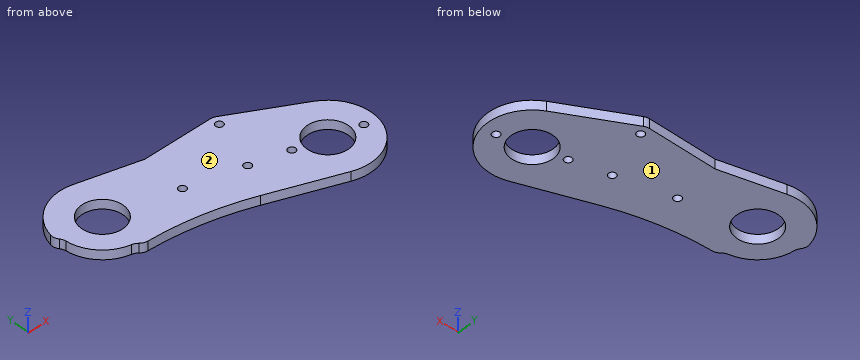
Autodesk Inventor part; units mm, degrees
ref_plane "YZ Plane" through (0, 0, 0) normal (1, 0, 0) x (0, 1, 0)
ref_plane "XZ Plane" through (0, 0, 0) normal (0, 1, 0) x (-1, 0, 0)
ref_plane "XY Plane" through (0, 0, 0) normal (0, 0, 1) x (1, 0, 0)
sketch "Sketch1" plane through (0, 0, 0) normal (0, 0, 1) x (1, 0, 0)
  circle A0 centre (71.842, 71.842) radius 50.8 construction
  circle A1 centre (-71.842, -71.842) radius 50.8 construction
  circle A2 centre (0, 0) radius 50.8 construction
  line L0 (-35.921, -35.921) -> (35.921, 35.921) construction
  line L1 (71.842, 71.842) -> (-71.842, -71.842) construction
  line L2 (-4.3707, 6.2419) -> (-4.3707, 50.6116) construction
  line L3 (-226.8798, -122.642) -> (638.5123, -122.642) construction
  circle A3 centre (147.8406, -65.492) radius 57.15 construction
  circle A4 centre (71.842, 71.842) radius 14.2621
  circle A5 centre (-71.842, -71.842) radius 14.2621
  circle A6 centre (-4.3707, 6.2419) radius 57.15 construction
  circle A7 centre (-71.842, -71.842) radius 30.1371 construction
  circle A8 centre (71.842, 71.842) radius 30.1371 construction
  circle A9 centre (-56.3286, 101.6778) radius 14.2621
  line L4 (-56.3286, 101.6778) -> (71.842, 71.842) construction
  circle A10 centre (71.842, 71.842) radius 14.3256 construction
  circle A11 centre (-71.842, -71.842) radius 14.3256 construction
  circle A12 centre (-78.675, 59.5778) radius 14.2621
  line L5 (-71.842, -71.842) -> (-78.675, 59.5778) construction
  circle A13 centre (-78.675, 59.5778) radius 23.8316 construction
  circle A14 centre (-56.3286, 101.6778) radius 23.8316 construction
  line L6 (14.7165, 60.1103) -> (61.7767, 43.4355)
  line L7 (-43.0113, -63.0652) -> (-59.0434, -10.4018)
  arc A15 (14.7165, 60.1103) -> (-59.0434, -10.4018) centre (-4.3707, 6.2419) ccw
  line L8 (-202.9564, 165.4321) -> (-177.9423, 161.0215)
  line L9 (-177.9423, 161.0215) -> (-204.4062, 10.9368) construction
  line L10 (-204.4062, 10.9368) -> (-229.4204, 15.3474) construction
  line L11 (-229.4204, 15.3474) -> (-202.9564, 165.4321) construction
  line L12 (-248.4004, -92.2937) -> (35.0702, -142.2772) construction
  line L13 (-201.8537, 171.6857) -> (161.0026, 107.7043) construction
  line L14 (-201.8537, 171.6857) -> (-248.4004, -92.2937) construction
  circle A16 centre (-147.7392, 94.6182) radius 31.75 construction
  line L15 (-77.4376, 35.7784) -> (-74.4797, -21.1106) construction
  line L16 (-190.4493, 163.2268) -> (-216.9133, 13.1421) construction
  line L17 (-193.206, 147.593) -> (-214.1566, 28.7759) construction
  circle A17 centre (-147.7392, 94.6182) radius 17.4625 construction
  circle A18 centre (-147.7392, 94.6182) radius 9.525
  circle A19 centre (-56.3286, 101.6778) radius 30.1816 construction
  line L18 (-202.9564, 165.4321) -> (-229.4204, 15.3474)
  arc A20 (61.7767, 43.4355) -> (78.6846, 101.1921) centre (71.842, 71.842) ccw
  arc A21 (-99.1524, -84.5852) -> (-43.0113, -63.0652) centre (-71.842, -71.842) ccw
  line L19 (-147.7392, 94.6182) -> (-131.3298, 100.5908) construction
  line L20 (-113.4287, 107.1063) -> (-182.0497, 82.1302) construction
  circle A22 centre (-182.0497, 82.1302) radius 4.7625 construction
  line L21 (0, 0) -> (-4.3707, 6.2419) construction
  circle A23 centre (71.842, 71.842) radius 28.6512 construction
  line L22 (62.334, 44.8145) -> (-61.0615, 88.2239) construction
  line L23 (75.2477, 100.2901) -> (-54.6333, 115.8388) construction
  line L24 (-177.9423, 161.0215) -> (78.6846, 101.1921)
  line L25 (-147.7392, 94.6182) -> (-125.7265, 22.8485) construction
  circle A24 centre (-125.7265, 22.8485) radius 31.75 construction
  circle A25 centre (-125.7265, 22.8485) radius 14.2621
  line L26 (-78.675, 59.5778) -> (-125.7265, 22.8485) construction
  circle A26 centre (-147.7392, 94.6182) radius 25.4 construction
  arc A27 (-99.1524, -84.5852) -> (-229.4204, 15.3474) centre (-260.2996, -159.7777) ccw
  circle A28 centre (-147.7392, 94.6182) radius 36.5125 construction
  line L27 (-180.8308, 110.0491) -> (-147.7392, 94.6182) construction
  arc A29 (-39.1085, 126.4648) -> (-49.6289, 131.1064) centre (-56.3286, 101.6778) ccw
  arc A30 (-38.1634, 52.3307) -> (-39.1085, 126.4648) centre (-65.0941, 89.0604) ccw
  arc A31 (14.7165, 60.1103) -> (-55.7287, 71.5022) centre (-51.7719, -127.535) ccw
  arc A32 (-49.6289, 131.1064) -> (-55.7287, 71.5022) centre (-56.3286, 101.6778) ccw
  line L28 (-10.7972, 91.0789) -> (26.3107, 82.4409) construction
  point P0 (-75.9587, 7.3339)
  point P1 (-203.6813, 88.1845)
  point P2 (-203.6813, 88.1845)
  point P3 (-144.7069, 111.8154)
  point P4 (-161.1163, 105.8429)
  point P5 (-164.1486, 88.6457)
  point P6 (-150.7715, 77.421)
  point P7 (-134.3622, 83.3936)
  point P8 (-123.871, 103.3056)
  point P9 (-143.3285, 119.6324)
  point P10 (-167.1967, 110.945)
  point P11 (-171.6074, 85.9309)
  point P12 (-152.1499, 69.6041)
  point P13 (-128.2817, 78.2914)
  point P14 (-160.2272, 128.9288)
  point P15 (-182.0497, 82.1302)
  point P16 (-135.2512, 60.3077)
  point P17 (-132.3084, 127.7098)
  point P18 (-163.1701, 61.5267)
  point P19 (-114.6476, 79.1874)
  point P20 (-49.4759, 131.0711)
  point P21 (7.7567, 86.7599)
  dimension "d7" = 101.6
  dimension "d18" = 47.6631
  dimension "d34" = 34.925
  dimension "d65" = 50.8
  dimension "d3" = 45
  dimension "d4" = 0
  dimension "d8" = 101.6
  dimension "d9" = 28.5242
  dimension "d10" = 101.6
  dimension "d11" = 114.3
  dimension "d12" = 114.3
  dimension "d13" = 15.875
  dimension "d14" = 15.875
  dimension "d15" = 131.5974
  dimension "d16" = 28.6512
  dimension "d17" = 131.5974
  dimension "d19" = 47.6631
  dimension "d22" = 25.4
  dimension "d23" = 152.4
  dimension "d26" = 268.0517
  dimension "d27" = 63.5
  dimension "d30" = 203.2
  dimension "d31" = 10
  dimension "d33" = 120.65
  dimension "d35" = 19.05
  dimension "d36" = 6.35
  dimension "d40" = 360
  dimension "d44" = 9.525
  dimension "d55" = 80
  dimension "d56" = 7.62
  dimension "d57" = 6.35
  dimension "d58" = 57.3024
  dimension "d59" = 63.5
  dimension "d60" = 75.0697
  dimension "d61" = 59.69
  dimension "d62" = 55
  dimension "d68" = 360
  dimension "d70" = 41.275
  dimension "d71" = 60
  dimension "d82" = 360
  dimension "d87" = 360
  dimension "d89" = 45
  dimension "d105" = 38.1
extrude "Extrusion1" add sketch "Sketch1" along normal blind 6.35 contours A29 A30 A31 A32 | A31 A30 A29 L24 A20 L6
hole "Hole1" at (-193.206, 147.593, 0) at (-203.6813, 88.1845, 0) at (-214.1566, 28.7759, 0) at (-131.3298, 100.5908, 0) at (-144.7069, 111.8154, 0) at (-161.1163, 105.8429, 0) at (-164.1486, 88.6457, 0) at (-150.7715, 77.421, 0) at (-134.3622, 83.3936, 0) at (-113.4287, 107.1063, 0) at (-182.0497, 82.1302, 0) at (-152.1499, 69.6041, 0) at (-171.6074, 85.9309, 0) at (-167.1967, 110.945, 0) at (-143.3285, 119.6324, 0) at (-123.871, 103.3056, 0) at (-128.2817, 78.2914, 0) at (-75.9587, 7.3339, 0) at (-180.8308, 110.0491, 0) at (-132.3084, 127.7098, 0) at (-114.6476, 79.1874, 0) at (-163.1701, 61.5267, 0) at (-10.7972, 91.0789, 0) at (26.3107, 82.4409, 0) direction (0, 0, 1) diameter 5.1054 end through all
sketch "Sketch2" plane through (0, 0, 6.35) normal (0, 0, 1) x (1, 0, 0)
  line L0 (78.6846, 101.1921) -> (-49.4759, 131.0711) construction
  circle A0 centre (-56.3286, 101.6778) radius 14.2621 construction
  line L1 (-76.7997, 106.4431) -> (-35.8574, 96.9125) construction
  line L2 (51.3709, 76.6074) -> (92.3132, 67.0767) construction
  line L3 (-56.3286, 101.6778) -> (71.842, 71.842) construction
  arc A1 (-49.4759, 131.0711) -> (-55.7287, 71.5022) centre (-56.3286, 101.6778) ccw
  arc A2 (14.7165, 60.1103) -> (-55.7287, 71.5022) centre (-51.7719, -127.535) ccw
  line L4 (14.7165, 60.1103) -> (61.7767, 43.4355)
  arc A3 (61.7767, 43.4355) -> (78.6846, 101.1921) centre (71.842, 71.842) ccw
  point P0 (0, 0)
hole "Hole2" at (92.3132, 67.0767, 6.35) at (51.3709, 76.6074, 6.35) direction (0, 0, -1) diameter 5.1054 end through all
sketch "Sketch3" plane through (0, 0, 6.35) normal (0, 0, 1) x (1, 0, 0)
  circle A0 centre (92.3132, 67.0767) radius 2.5527 construction
  circle A1 centre (51.3709, 76.6074) radius 2.5527 construction
  arc A2 (14.7165, 60.1103) -> (-55.7287, 71.5022) centre (-51.7719, -127.535) ccw construction
  line L0 (14.7165, 60.1103) -> (61.7767, 43.4355) construction
  arc A3 (61.7767, 43.4355) -> (78.6846, 101.1921) centre (71.842, 71.842) ccw construction
  line L1 (78.6846, 101.1921) -> (-49.4759, 131.0711) construction
  arc A4 (-49.4759, 131.0711) -> (-55.7287, 71.5022) centre (-56.3286, 101.6778) ccw construction
  circle A5 centre (71.842, 71.842) radius 14.2621 construction
  circle A6 centre (-56.3286, 101.6778) radius 14.2621 construction
  circle A7 centre (71.842, 71.842) radius 14.2621 construction
  line L2 (-56.3286, 101.6778) -> (71.842, 71.842) construction
  line L3 (30.0957, 81.5598) -> (38.3306, 116.936) construction
  line L4 (41.3443, 122.5253) -> (86.1452, 98.3687)
  arc A8 (61.7767, 43.4355) -> (78.6846, 101.1921) centre (71.842, 71.842) ccw construction
  line L5 (78.6846, 101.1921) -> (-49.4759, 131.0711) construction
  arc A9 (86.1452, 98.3687) -> (78.6846, 101.1921) centre (71.842, 71.842) ccw
  arc A10 (41.3443, 122.5253) -> (38.0994, 123.2818) centre (38.3306, 116.936) ccw
  arc A11 (36.8909, 110.7514) -> (36.9386, 110.7405) centre (38.3306, 116.936) ccw
  line L6 (38.0994, 123.2818) -> (-8.7442, 121.575)
  line L7 (78.6846, 101.1921) -> (-8.7442, 121.575)
  point P0 (0, 0)
  dimension "d90" = 42.8625
  dimension "d91" = 36.322
  dimension "d102" = 6.35
  dimension "d103" = 15.21
  dimension "d104" = 15.21
extrude "Extrusion2" add sketch "Sketch3" against normal up to surface (6.35 mm away)
sketch "Sketch4" plane through (0, 0, 6.35) normal (0, 0, 1) x (1, 0, 0)
  arc A0 (41.3443, 122.5253) -> (38.0994, 123.2818) centre (38.3306, 116.936) ccw construction
  point P0 (0, 0)
hole "Hole3" at (38.3306, 116.936, 6.35) direction (0, 0, -1) diameter 5.1054 end through all
sketch "Sketch5" plane through (0, 0, 6.35) normal (0, 0, 1) x (1, 0, 0)
  circle A0 centre (38.3306, 116.936) radius 2.5527 construction
  circle A1 centre (92.3132, 67.0767) radius 2.5527 construction
  circle A2 centre (51.3709, 76.6074) radius 2.5527 construction
  circle A3 centre (-10.7972, 91.0789) radius 2.5527 construction
  circle A4 centre (26.3107, 82.4409) radius 2.5527 construction
  arc A5 (14.7165, 60.1103) -> (-55.7287, 71.5022) centre (-51.7719, -127.535) ccw construction
  line L0 (14.7165, 60.1103) -> (61.7767, 43.4355) construction
  arc A6 (61.7767, 43.4355) -> (86.1452, 98.3687) centre (71.842, 71.842) ccw construction
  line L1 (86.1452, 98.3687) -> (41.3443, 122.5253) construction
  arc A7 (41.3443, 122.5253) -> (38.0994, 123.2818) centre (38.3306, 116.936) ccw construction
  line L2 (38.0994, 123.2818) -> (-8.7442, 121.575) construction
  line L3 (-8.7442, 121.575) -> (-49.4759, 131.0711) construction
  arc A8 (-49.4759, 131.0711) -> (-55.7287, 71.5022) centre (-56.3286, 101.6778) ccw
  circle A9 centre (71.842, 71.842) radius 14.2621 construction
  circle A10 centre (-56.3286, 101.6778) radius 14.2621 construction
  arc A11 (-49.4759, 131.0711) -> (-55.7287, 71.5022) centre (-56.3286, 101.6778) ccw construction
  line L4 (-86.3452, 104.8286) -> (-83.1507, 104.8286)
  arc A12 (14.7165, 60.1103) -> (-55.7287, 71.5022) centre (-51.7719, -127.535) ccw construction
  line L5 (-55.7287, 71.5022) -> (-55.7287, 74.6779)
  arc A13 (-83.1507, 104.8286) -> (-55.7287, 74.6779) centre (-56.3286, 101.6778) ccw
  point P0 (0, 0)
  dimension "d114" = 3.175
extrude "Extrusion3" cut sketch "Sketch5" against normal through all
fillet "Fillet1" radius 6.604 4 edges at (-83.1507, 104.8286, 3.175) (-86.3452, 104.8286, 3.175) (-55.7287, 74.6779, 3.175) (-55.7287, 71.5022, 3.175)
properties part number "GP10-002" material "Polycarbonate, Smoke"
Part model, mm, in its own coordinate system. Face numbers are marked on the shaded views. Give positions to 0.01 mm unless a question says otherwise; leave off trailing zeros. Order: outer loops, then holes, each group sorted by start corner. A loop starts at its lowest first (then second) coordinate and runs counter-clockwise, first axis right, second up. Notation, with made-up numbers: (88.25, -16) -> (123.25, -16) arc R37 ccw to (123.25, 21) -> close; hole circle Ø3 at (29, 42.5). An arc over 180 degrees is marked (long way). Use one line per item in the form item = value.
(1) Drill centre lines: line 1 (Y direction, x = 36, z = 3.5); line 2 (Y direction, x = -46.5, z = 1.25); line 3 (X direction, y = 118.5, z = 5.75). Where is each one in solid material? Low to high. Write a range as from..to.
Solution:
line_1 = 52.57..115.89, 117.98..123.21
line_2 = 71.47..91.34, 112.01..130.38
line_3 = -81.39..36.31, 40.35..48.81
(2) Flat gauge pins, fed straight in: P1, Ø4, axis at x = -13, y = 64.5, coming from the +Z side; P2, Ø1, axis at y = 93, z = 3.5, coming from the -X side. Where does each tip first touch, or does it go through?
Solution:
P1 = through
P2 = -82.07
(3) Pull direction Z, two halves, no side cores. Call the marked faces 1 and 2: +Z half, -Z half, draft (parallel to the pull), parting line (faces both ways), or undercut.
Solution:
face_1 = -Z half
face_2 = +Z half
(4) Saw through at A-A (x = -66.5). Write the cut outline in (y, z).
Solution:
outline = (76.66, 0) -> (91.68, 0) -> (91.68, 6.35) -> (76.66, 6.35) -> close; (111.68, 0) -> (130.09, 0) -> (130.09, 6.35) -> (111.68, 6.35) -> close
(5) Saw through at D-D (y = 52). Write the cut outline in (x, z), then the cut area to 3 significant figures.
Solution:
outline = (37.61, 0) -> (94.53, 0) -> (94.53, 6.35) -> (37.61, 6.35) -> close
area = 361 mm²
(6) Saw through at C-C (x = 68). Write the cut outline in (y, z).
Solution:
outline = (41.95, 0) -> (58.11, 0) -> (58.11, 6.35) -> (41.95, 6.35) -> close; (85.58, 0) -> (108.15, 0) -> (108.15, 6.35) -> (85.58, 6.35) -> close
(7) Saw through at B-B (z = 2). Write the cut outline in (x, y) (1 decimal), then the cut area to 3 significant figures.
Solution:
outline = (-85.7, 108.7) arc R6.6 ccw to (-84.6, 103.2) arc R6.6 cw to (-83.3, 99.7) arc R27 ccw to (-60.6, 75) arc R6.6 cw to (-57.1, 73.3) arc R6.6 ccw to (-52.6, 71.5) arc R199.1 cw to (14.7, 60.1) -> (61.8, 43.4) arc R30.1 ccw to (86.1, 98.4) -> (41.3, 122.5) arc R6.3 ccw to (38.1, 123.3) -> (-8.7, 121.6) -> (-49.6, 131.1) arc R30.2 ccw to start; hole circle Ø28.5 at (-56.3, 101.7); hole circle Ø5.1 at (-10.8, 91.1); hole circle Ø5.1 at (26.3, 82.4); hole circle Ø5.1 at (38.3, 116.9); hole circle Ø5.1 at (51.4, 76.6); hole circle Ø28.5 at (71.8, 71.8); hole circle Ø5.1 at (92.3, 67.1)
area = 9,320 mm²
